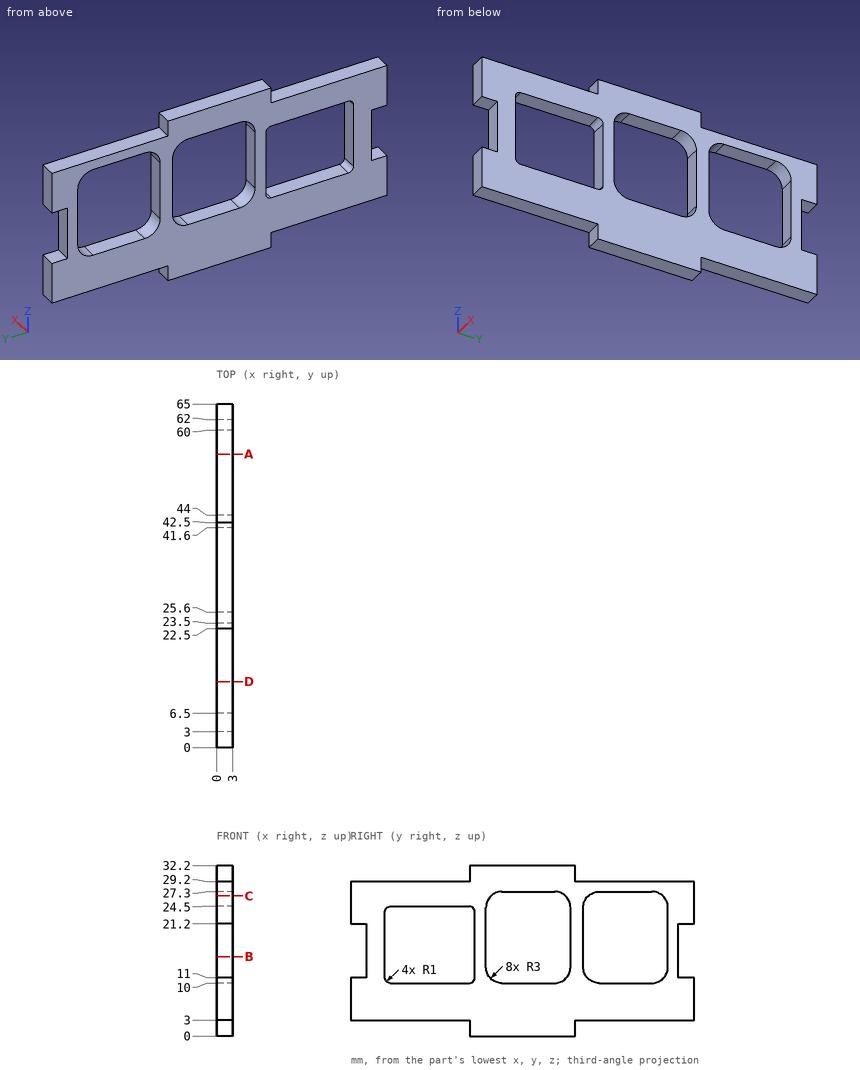
Job drawing, mm, ordinate dimensions from the low corner. One solid piece. Coordinates: 2 decimals unless noted, no trailing zeros. Loops run counter-clockwise (first coordinate to the right, second up) from the corner with the lowest first, then second, coordinate; pieces in that order, holes last. Notation, with made-up numbers: (78.25, 87.25) - (135.25, 87.25) arc R17 cw to (135.25, 92.25) - close; hole circle Ø5 at (69.25, -24.75). An arc over 180 degrees is marked (long way). Write item = value, one per line. Start each with the question number.
Q1. Drill centre lines: L1, parallel to Y at x = 0.85, z = 18; L2, parallel to Y at x = 1.4, z = 23.5; L3, parallel to Z at x = 0.9, y = 20. Where is each one in solid material? Low to high.
Q2. Cut at A-A, the plane y = 55.5. List the corners of the cut face in (x, z), then the cut area to 3 significant figures.
Q3. Cut at D-D, the plane y = 12.5. List the corners of the cut face in (x, z), then the cut area to 3 significant figures.
Q4. Flat gauge pins, fed straight in: pin 1 Ø0.9 at (x, y) = (2, 5.5) entering from -Z; pin 2 Ø1.5 at (x, z) = (0.5, 16) entering from -Y; pin 3 Ø0.9 at (x, z) = (2, 17) entering from +Y. Where does each tip first touch, or does it go through?
Q5. Cut at C-C, the plane z = 26.5. List the corners of the cut face in (x, y), then the cut area to 3 significant figures.
Q6. Cut at B-B, the plane z = 15. List the corners of the cut face in (x, y), then the cut area to 3 significant figures.
Computed:
q1.L1 = 3 to 6.5, 23.5 to 25.6, 41.6 to 44, 60 to 62
q1.L2 = 0 to 6.5, 23.5 to 25.6, 41.6 to 44, 60 to 65
q1.L3 = 3 to 10, 24.5 to 29.2
q2.outline = (0, 3) - (3, 3) - (3, 10) - (0, 10) - close; (0, 27.3) - (3, 27.3) - (3, 29.2) - (0, 29.2) - close
q2.area = 26.7 mm²
q3.outline = (0, 3) - (3, 3) - (3, 10) - (0, 10) - close; (0, 24.5) - (3, 24.5) - (3, 29.2) - (0, 29.2) - close
q3.area = 35.1 mm²
q4.pin_1 = 3
q4.pin_2 = 3
q4.pin_3 = 62
q5.outline = (0, 0) - (3, 0) - (3, 26.56) - (0, 26.56) - close; (0, 40.64) - (3, 40.64) - (3, 44.96) - (0, 44.96) - close; (0, 59.04) - (3, 59.04) - (3, 65) - (0, 65) - close
q5.area = 111 mm²
q6.outline = (0, 3) - (3, 3) - (3, 6.5) - (0, 6.5) - close; (0, 23.5) - (3, 23.5) - (3, 25.6) - (0, 25.6) - close; (0, 41.6) - (3, 41.6) - (3, 44) - (0, 44) - close; (0, 60) - (3, 60) - (3, 62) - (0, 62) - close
q6.area = 30.0 mm²
